Job drawing, mm, ordinate dimensions from the low corner. One solid piece. Coordinates: 2 decimals unless noted, no trailing zeros. Order: outer loops, then holes, each group sorted by start corner. A loop starts at its lowest first (then second) coordinate and runs counter-clockwise, first axis right, second up. Notation, with made-up numbers: (48, 61) - (80, 61) arc R35 ccw to (80, 93) - close; hole circle Ø1 at (17, -32). An arc over 180 degrees is marked (long way). Use a Markdown table: item, result. Add a question column.
1) Saw through at A-A on x = 147.5. List the corners of the cut face in (y, z).
2) Wall check: L1, parallel to Y at x = 147.5, z = 1.6; L2, parallel to X at y = 7.25, z = 0.4; L3, parallel to X at y = 5, z = 1.2. Give the ranges that are in metal, low to high. Write a range as [from, to].
3) Drop flat-ended pins along their axis: P1, Ø4.5, axis at x = 147.5, y = 6, coming from the -Z side; P2, Ø0.8, axis at y = 6, z = 0.5, coming from the +X side. Give the stop position or say it passes through.
4) Saw through at B-B on y = 6. List the corners of the cut face in (x, z).
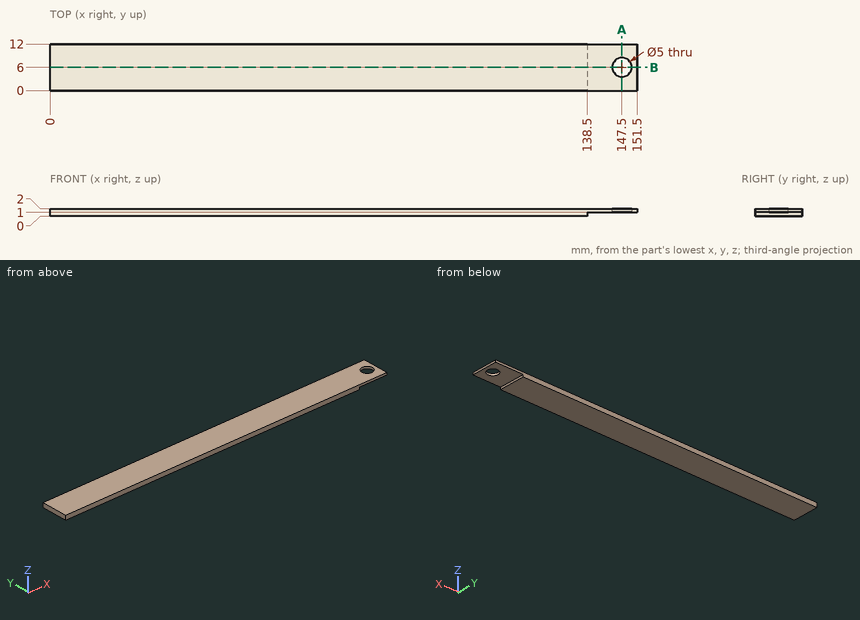
Results are:
| question | item | result |
|---|---|---|
| 1 | outline | (0, 1) - (3.5, 1) - (3.5, 2) - (0, 2) - close; (8.5, 1) - (12, 1) - (12, 2) - (8.5, 2) - close |
| 2 | L1 | [0, 3.5], [8.5, 12] |
| 2 | L2 | [0, 138.5] |
| 2 | L3 | [0, 145.21], [149.79, 151.5] |
| 3 | P1 | through |
| 3 | P2 | x = 138.5 |
| 4 | outline | (0, 0) - (138.5, 0) - (138.5, 1) - (145, 1) - (145, 2) - (0, 2) - close; (150, 1) - (151.5, 1) - (151.5, 2) - (150, 2) - close |
